from build123d import *

# Parameters (mm, degrees)
SKETCH1_R           = 2.75
SKETCH1_R_2         = 1.4
BOSS_EXTRUDE1_DEPTH = 6.6
SKETCH2_R           = 4.25
BOSS_EXTRUDE2_DEPTH = 1.1
SKETCH3_R           = 2.6
SKETCH3_R_2         = 1.35
BOSS_EXTRUDE3_DEPTH = 1
FILLET1_R           = 0.6


with BuildPart() as part:
    # Sketch1 → Boss-Extrude1 (new body)
    with BuildSketch(Plane(origin=(0, 0, 0), x_dir=(1, 0, 0), z_dir=(0, 1, 0))):
        Circle(SKETCH1_R)
        Circle(SKETCH1_R_2, mode=Mode.SUBTRACT)
    extrude(amount=BOSS_EXTRUDE1_DEPTH)

    # Sketch2 → Boss-Extrude2 (add)
    with BuildSketch(Plane(origin=(0, 6.6, 0), x_dir=(1, 0, 0), z_dir=(0, 1, 0))):
        Circle(SKETCH2_R)
    extrude(amount=BOSS_EXTRUDE2_DEPTH)

    # Sketch3 → Boss-Extrude3 (add)
    with BuildSketch(Plane(origin=(0, 7.7, 0), x_dir=(1, 0, 0), z_dir=(0, 1, 0))):
        Circle(SKETCH3_R)
        Circle(SKETCH3_R_2, mode=Mode.SUBTRACT)
    extrude(amount=BOSS_EXTRUDE3_DEPTH)

    # Fillet1
    fillet1_edges = [part.edges().sort_by_distance(p)[0] for p in [
        (-2.6, 8.7, 0),
        (-1.35, 8.7, 0),
        (-4.25, 7.7, 0),
    ]]
    fillet(fillet1_edges, radius=FILLET1_R)


solid = part.part
Verification items for the finished model (mm, model axes). A direction names the side the tool comes from. Give positions to 0.01 mm unless a question says otherwise; leave off trailing zeros. Write each loop counter-clockwise with the first axis right and the second up, starting at its lowest first coordinate (ties: lowest second). Pieces come first, ordered by that corner, then holes. Notation, with made-up numbers: M 23,59.25 L 69,59.25 A25 cw 69,87.25 Z; hole C 47.5,53.5 d3. An arc over 180 degrees is marked long. Write item = value, one per line.
(1) Sectioned sample at A-A (x = 0). Record the cut outline in (y, z), then the cut area to 3 significant figures.
Found:
outline = M 0,-2.75 L 6.6,-2.75 L 6.6,-4.25 L 7.1,-4.25 A0.6 ccw 7.7,-3.65 L 7.7,-2.6 L 8.1,-2.6 A0.6 ccw 8.7,-2 L 8.7,-1.95 A0.6 ccw 8.1,-1.35 L 7.7,-1.35 L 7.7,1.35 L 8.1,1.35 A0.6 ccw 8.7,1.95 L 8.7,2 A0.6 ccw 8.1,2.6 L 7.7,2.6 L 7.7,3.65 A0.6 ccw 7.1,4.25 L 6.6,4.25 L 6.6,2.75 L 0,2.75 L 0,1.4 L 6.6,1.4 L 6.6,-1.4 L 0,-1.4 Z
area = 29.2 mm2
(2) Material ranges on line 1 (Z direction, x = 0, y = 2.25); line 2 (Z direction, x = 0, y = 7.9), recorded low to high.
Found:
line_1 = -2.75 to -1.4, 1.4 to 2.75
line_2 = -2.6 to -1.35, 1.35 to 2.6
(3) Go/stop test with flat-tipped pins: pin 1 Ø1.7 at (x, z) = (0, 0) entering from +Y; pin 2 Ø5 at (x, y) = (-3.5, 2) entering from +Z; pin 3 Ø2 at (x, z) = (-1, 2) entering from +Y; pin 4 Ø3 at (x, y) = (0.5, 3) entering from +Z. Record where each tip stops, or that it passes through.
Found:
pin_1 = 7.7
pin_2 = 2.56
pin_3 = 8.7
pin_4 = 2.75
(4) Access from +Z, -Z, +X, -X, +Y, -Y to the whole of each face (thin tool, end or side, straight path). Record for faces 4 (the face through (1.2, 0, 1.2)), 5 (the face through (0, 6.6, 0)), 6 (the face through (-0.338, 7.897, -2.578)).
Found:
face_4 = +Z, -Z, +X, -X, -Y
face_5 = -Y
face_6 = +Y
(5) Draft check along X on faces 1 (the face through (2.285, 6.846, -3.584)), 2 (the face through (0, 7.7, 0)), 3 (the face through (0, 6.6, 3)). Enter one of: released by +X, released by -X, zero draft, split by the parting line, or undercut.
Found:
face_1 = split by the parting line
face_2 = undercut
face_3 = zero draft
(6) Sectioned sample at B-B (y = 2). Record the cut outline in (x, z), then the cut area to 3 significant figures.
Found:
outline = C 0,0 d5.5; hole C 0,0 d2.8
area = 17.6 mm2
